Geometry check sheet. Reference: drawing and pictorial views, mm from the part's lowest x, y, z. A direction names the side the tool comes from. Give positions to 0.01 mm unless a question says otherwise; leave off trailing zeros. Answer in a Markdown table with one row per item.
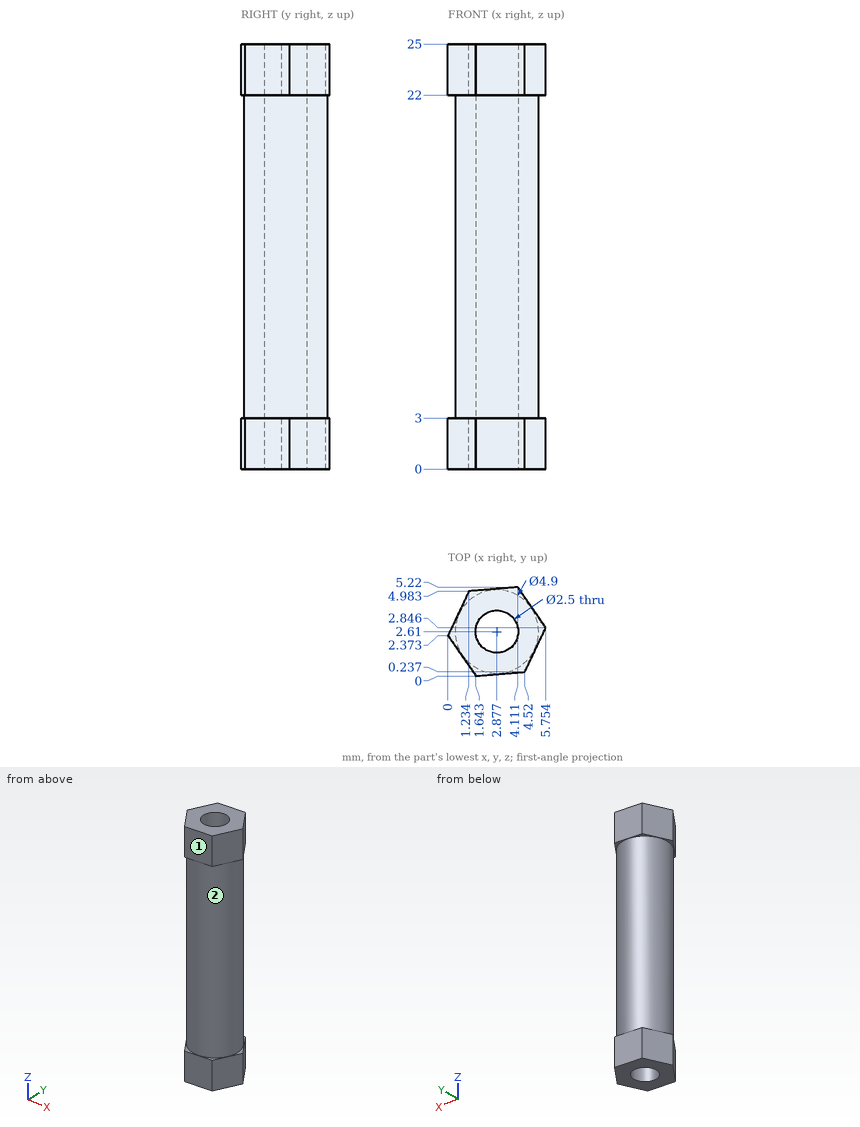
(1) Access from +Z, -Z, +X, -X, +Y, -Y to the whole of each face (thin tool, end or side, straight path). Record for the marked faces 1 and 2.
Geometry says:
| item | result |
|---|---|
| face 1 | +Z, -Z, +X, -Y |
| face 2 | none |
(2) Gauge pin test, flat end, axial feed: P1, Ø2, axis at y = 3, z = 2.5, coming from the +X side. Record the tip position at first contact, or that the pin passes through.
Geometry says:
| item | result |
|---|---|
| P1 | x = 5.75 |
(3) Thickness scan on L1, parallel to X at y = 2.7, z = 8.75 (1 decimal); L2, parallel to X at y = 2.35, z = 16 (1 decimal); L3, parallel to Y at x = 3.5, z = 17.5 (1 decimal). Record the ranges inside material, lowest first.
Geometry says:
| item | result |
|---|---|
| L1 | 0.4 to 1.6, 4.1 to 5.3 |
| L2 | 0.4 to 1.7, 4.1 to 5.3 |
| L3 | 0.2 to 1.5, 3.7 to 5 |
